```python
from build123d import *

# Parameters (mm, degrees)
ESQUISSE1_W             = 7.08
ESQUISSE1_H             = 3.88
BOSS_EXTRU_1_DEPTH      = 2.05
ESQUISSE3_W             = 5.163612044
ESQUISSE3_H             = 0.48908098
ENL_V_MAT_EXTRU_1_DEPTH = 2.05
ESQUISSE4_W             = 5.163612044
ESQUISSE4_H             = 3.39091902
ENL_V_MAT_EXTRU_2_DEPTH = 0.1
ESQUISSE5_W             = 5.163612044
ESQUISSE5_H             = 3.39091902
ENL_V_MAT_EXTRU_3_DEPTH = 0.1
CONG_1_R                = 0.25


with BuildPart() as part:
    # Esquisse1 → Boss.-Extru.1 (new body)
    with BuildSketch(Plane.XY):
        Rectangle(ESQUISSE1_W, ESQUISSE1_H)
    extrude(amount=BOSS_EXTRU_1_DEPTH)

    # Esquisse3 → Enlèv. mat.-Extru.1 (cut)
    with BuildSketch(Plane.XY.offset(2.05)):
        with Locations((0, 1.94)):
            Rectangle(ESQUISSE3_W, ESQUISSE3_H)
        with Locations((0, -1.94)):
            Rectangle(ESQUISSE3_W, ESQUISSE3_H)
    extrude(amount=-ENL_V_MAT_EXTRU_1_DEPTH, mode=Mode.SUBTRACT)

    # Esquisse4 → Enlèv. mat.-Extru.2 (cut)
    with BuildSketch(Plane.XY.offset(2.05)):
        Rectangle(ESQUISSE4_W, ESQUISSE4_H)
    extrude(amount=-ENL_V_MAT_EXTRU_2_DEPTH, mode=Mode.SUBTRACT)

    # Esquisse5 → Enlèv. mat.-Extru.3 (cut)
    with BuildSketch(Plane(origin=(0, 0, 0), x_dir=(-1, 0, 0), z_dir=(0, 0, -1))):
        Rectangle(ESQUISSE5_W, ESQUISSE5_H)
    extrude(amount=-ENL_V_MAT_EXTRU_3_DEPTH, mode=Mode.SUBTRACT)

    # Congé1
    cong_1_edges = [part.edges().sort_by_distance(p)[0] for p in [
        (-3.54, 0, 2.05),
        (3.54, 0, 2.05),
        (-3.54, 0, 0),
        (3.54, 0, 0),
        (3.54, -1.94, 1.025),
        (-3.54, -1.94, 1.025),
        (-3.54, 1.94, 1.025),
        (3.54, 1.94, 1.025),
    ]]
    fillet(cong_1_edges, radius=CONG_1_R)


solid = part.part
```
Source: CAD feature listing. Evaluate the final solid. Frame: model axes, mm. A direction names the side the tool comes from. Give positions to 0.01 mm unless a question says otherwise; leave off trailing zeros. Write each loop counter-clockwise with the first axis right and the second up, starting at its lowest first coordinate (ties: lowest second). Pieces come first, ordered by that corner, then holes.
1. Access query for faces 1 (the face through (0, 0, 1.95)), 2 (the face through (0, -1.695, 1)), 3 (the face through (0, 1.695, 1)). Directions: +Z, -Z, +X, -X, +Y, -Y. A direction counts if a zero-diameter tool reaches every point of the face in a straight line with its end or side. Return the directions, or none.
2. Pull-direction query (X, two-part tool) for faces 4 (the face through (-3.54, 0, 1)), 5 (the face through (0, 0, 0.1)), 6 (the face through (3.54, 0, 1)); classes: +X half, -X half, draft (parallel to the pull), parting line (faces both ways), or undercut.
3. First-contact query: pin 1 (1 mm diameter, centred on x = -1, z = 0.5, fed in from +Y); pin 2 (1.5 mm diameter, centred on x = -0.5, y = 0.5, fed in from -Z); pin 3 (1 mm diameter, centred on x = -0.5, y = 1, fed in from +Z). Flat tips, straight axial feed; report the tip coordinate or a pass-through.
4. Section query A-A (y = -1.6). Return the cut outline in (x, z).
5. Material intervals for line 1 along Y through (x, z) = (1.75, 0.75); line 2 along Z through (x, y) = (1, 0.2); line 3 along X through (y, z) = (1.75, 0.65), sorted ascending.
6. Section query B-B (z = 1.6). Return the cut outline in (x, y).
7. Section query C-C (x = -0.25). Return the cut outline in (y, z).
Output values:
1. face 1: +Z, +Y, -Y
1. face 2: +Z, -Z, -Y
1. face 3: +Z, -Z, +Y
2. face 4: -X half
2. face 5: undercut
2. face 6: +X half
3. pin 1: stops at y = 1.7
3. pin 2: stops at z = 0.1
3. pin 3: stops at z = 1.95
4. outline: (-3.54, 0.25) arc R0.25 ccw to (-3.29, 0) - (-2.58, 0) - (-2.58, 0.1) - (2.58, 0.1) - (2.58, 0) - (3.29, 0) arc R0.25 ccw to (3.54, 0.25) - (3.54, 1.8) arc R0.25 ccw to (3.29, 2.05) - (2.58, 2.05) - (2.58, 1.95) - (-2.58, 1.95) - (-2.58, 2.05) - (-3.29, 2.05) arc R0.25 ccw to (-3.54, 1.8) - close
5. line 1: y = -1.7 to 1.7
5. line 2: z = 0.1 to 1.95
5. line 3: x = -3.53 to -2.58, 2.58 to 3.53
6. outline: (-3.54, -1.69) arc R0.25 ccw to (-3.29, -1.94) - (-2.58, -1.94) - (-2.58, -1.7) - (2.58, -1.7) - (2.58, -1.94) - (3.29, -1.94) arc R0.25 ccw to (3.54, -1.69) - (3.54, 1.69) arc R0.25 ccw to (3.29, 1.94) - (2.58, 1.94) - (2.58, 1.7) - (-2.58, 1.7) - (-2.58, 1.94) - (-3.29, 1.94) arc R0.25 ccw to (-3.54, 1.69) - close
7. outline: (-1.7, 0.1) - (1.7, 0.1) - (1.7, 1.95) - (-1.7, 1.95) - close
